Could you check a few things on this model? Use its own coordinates, in mm. Face numbers are marked on the shaded views. A direction names the side the tool comes from. Give positions to 0.01 mm unless a question says otherwise; leave off trailing zeros. Loops run counter-clockwise (first coordinate to the right, second up) from the corner with the lowest first, then second, coordinate; pieces in that order, holes last. Notation, with made-up numbers: (73, 10) -> (99, 10) arc R21 ccw to (99, 39) -> close; hole circle Ø4 at (33, -5.75). An arc over 180 degrees is marked (long way). Write item = value, one per line. Start each with the question number.
1) On a 3-axis mill with a long thin cutter (end or side, diameter ignored), from which of +Z, -Z, +X, -X, +Y, -Y can I reach the whole of each face in a straight line? I mean the marked faces 1, 2 and 3. Say none if no direction works.
2) I want a section at C-C (y = 30.5). List the corners of the cut face in (x, z) for me, and give its area (3 significant figures).
3) If we mould it in two halves opening along Z, with no side actions, what happens to the marked faces 4, 5 and 6? For each: +Z half, -Z half, draft (parallel to the pull), parting line (faces both ways), or undercut.
4) I need wall thicknesses on probe 1 along Y at (x, z) = (0, 15); probe 2 along X at (y, z) = (45.5, -12); probe 3 along Z at (x, y) = (-24.5, 63.5). Which ranges of each line are inside material? Lowest first, please. Write a range as from..to.
5) I want a section at B-B (z = 0). List the corners of the cut face in (x, y) for me, and give its area (3 significant figures).
6) I want a section at A-A (x = 0). List the corners of the cut face in (y, z) for me, and give its area (3 significant figures).
7) I'm going to push flat-ended pins straight in: pin 1 Ø3 at (x, z) = (-40, 11.5) entering from -Y; pin 2 Ø8 at (x, y) = (-15, 66) entering from +Z; pin 3 Ø12 at (y, z) = (33, 5.5) entering from +X; pin 4 Ø12 at (y, z) = (53.5, -6.5) entering from -X. Where does each tip first touch, or does it pass through?
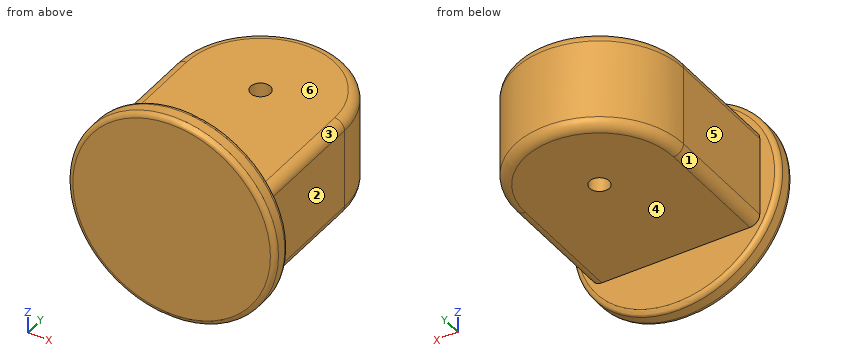
Autodesk Inventor part; units mm, degrees
ref_plane "YZ Plane" through (0, 0, 0) normal (1, 0, 0) x (0, 1, 0)
ref_plane "XZ Plane" through (0, 0, 0) normal (0, 1, 0) x (-1, 0, 0)
ref_plane "XY Plane" through (0, 0, 0) normal (0, 0, 1) x (1, 0, 0)
sketch "Sketch1" plane through (0, 0, 0) normal (0, 0, 1) x (1, 0, 0)
  line L0 (0, 0) -> (50, 0)
  line L1 (52.5, 2.5) -> (52.5, 7.5)
  line L2 (50, 10) -> (0, 10)
  line L3 (0, 10) -> (0, 0)
  arc A0 (52.5, 7.5) -> (50, 10) centre (50, 7.5) ccw
  arc A1 (50, 0) -> (52.5, 2.5) centre (50, 2.5) ccw
  point P0 (52.5, 0)
  point P1 (52.5, 10)
  dimension "d0" = 105
  dimension "d1" = 10
  dimension "d2" = 2.5
revolve "Revolution1" add sketch "Sketch1" angle 360 about axis through (0, 10, 0) along (0, -1, 0)
sketch "Sketch2" plane through (0, 0, 0) normal (0, 0, 1) x (1, 0, 0)
  line L0 (-52.5, 2.5) -> (52.5, 2.5)
  line L1 (-50, 0) -> (50, 0)
  line L2 (-50, 10) -> (50, 10)
  line L3 (-52.5, 7.5) -> (52.5, 7.5)
  line L4 (-52.5, 7.5) -> (52.5, 7.5)
  line L5 (-52.5, 2.5) -> (52.5, 2.5)
  line L6 (-42.5, 10) -> (42.5, 10)
  line L7 (42.5, 10) -> (42.5, 70.7)
  line L8 (42.5, 70.7) -> (-42.5, 70.7) construction
  line L9 (-42.5, 70.7) -> (-42.5, 10)
  line L10 (0, 70.7) -> (0, 10) construction
  line L11 (-50, 10) -> (50, 10)
  arc A0 (42.5, 70.7) -> (-42.5, 70.7) centre (0, 70.7) ccw
  circle A1 centre (0, 70.7) radius 5
  point P0 (0, 0)
  point P1 (0, 0)
  dimension "d4" = 85
  dimension "d5" = 70.7
  dimension "d9" = 10
extrude "Extrusion1" add sketch "Sketch2" along normal mid plane 50
fillet "Fillet1" radius 5 6 edges at (-42.5, 40.35, 25) (42.5, 40.35, 25) (0, 113.2, 25) (42.5, 40.35, -25) (-42.5, 40.35, -25) (0, 113.2, -25)
properties part number "Base2"
Answer list:
q1.face_1 = -Z, -X, +Y
q1.face_2 = +Z, -Z, +X, +Y
q1.face_3 = +Z, +X, +Y
q2.outline = (-42.5, -20) arc R5 ccw to (-37.5, -25) -> (37.5, -25) arc R5 ccw to (42.5, -20) -> (42.5, 20) arc R5 ccw to (37.5, 25) -> (-37.5, 25) arc R5 ccw to (-42.5, 20) -> close
q2.area = 4,230 mm^2
q3.face_4 = -Z half
q3.face_5 = draft
q3.face_6 = +Z half
q4.probe_1 = 0..65.7, 75.7..113.2
q4.probe_2 = -42.5..42.5
q4.probe_3 = -25..25
q5.outline = (-52.5, 2.5) arc R2.5 ccw to (-50, 0) -> (50, 0) arc R2.5 ccw to (52.5, 2.5) -> (52.5, 7.5) arc R2.5 ccw to (50, 10) -> (42.5, 10) -> (42.5, 70.7) arc R42.5 ccw to (-42.5, 70.7) -> (-42.5, 10) -> (-50, 10) arc R2.5 ccw to (-52.5, 7.5) -> close; hole circle Ø10 at (0, 70.7)
q5.area = 8,960 mm^2
q6.outline = (0, -50) arc R2.5 ccw to (2.5, -52.5) -> (7.5, -52.5) arc R2.5 ccw to (10, -50) -> (10, -25) -> (65.7, -25) -> (65.7, 25) -> (10, 25) -> (10, 50) arc R2.5 ccw to (7.5, 52.5) -> (2.5, 52.5) arc R2.5 ccw to (0, 50) -> close; (75.7, -25) -> (108.2, -25) arc R5 ccw to (113.2, -20) -> (113.2, 20) arc R5 ccw to (108.2, 25) -> (75.7, 25) -> close
q6.area = 5,690 mm^2
q7.pin_1 = 0
q7.pin_2 = 25
q7.pin_3 = 42.5
q7.pin_4 = -42.5
